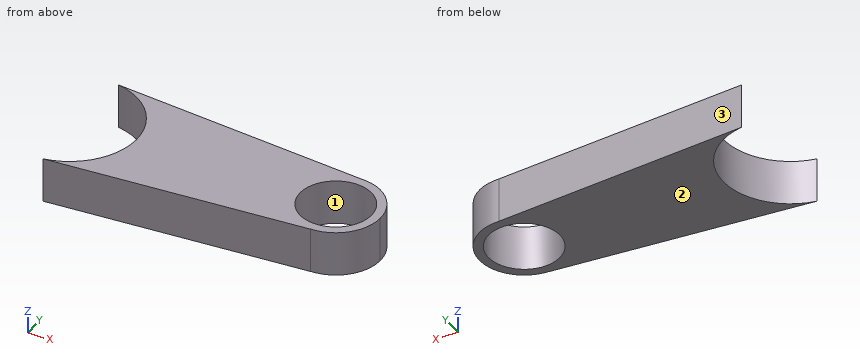
from build123d import *

# Parameters (mm, degrees)
F1_DEPTH = 5
F3_D     = 8


with BuildPart() as f1:
    # F0 (on Top) → F1 (new body)
    with BuildSketch(Plane.XY):
        with BuildLine():
            ThreePointArc((14.5967810947, -5), (18.1323150007, -3.5355339059), (19.5967810947, 0))
            ThreePointArc((19.5967810947, 0), (18.1323150007, 3.5355339059), (14.5967810947, 5))
            Line((14.5967810947, 5), (14.5967810947, 0))
            Line((14.5967810947, 0), (14.5967810947, -5))
        make_face()
        with BuildLine():
            Line((14.5967810947, 0), (14.5967810947, 5))
            ThreePointArc((14.5967810947, 5), (9.5967810947, 0), (14.5967810947, -5))
            Line((14.5967810947, -5), (14.5967810947, 0))
        make_face()
        with BuildLine():
            ThreePointArc((14.5967810947, -5), (9.5967810947, 0), (14.5967810947, 5))
            Line((14.5967810947, 5), (-14.1023044895, 7.3961588722))
            ThreePointArc((-14.1023044895, 7.3961588722), (-9.6198593647, 4.8436616619), (-7.8460222776, 0))
            ThreePointArc((-7.8460222776, 0), (-9.6226170145, -4.8469198667), (-14.110724196, -7.39756978))
            Line((-14.110724196, -7.39756978), (14.5967810947, -5.0171596368))
            Line((14.5967810947, -5.0171596368), (14.5967810947, -5))
        make_face()
    extrude(amount=F1_DEPTH)

    # F3 (through all)
    with Locations(Plane(origin=(0, 0, 0), x_dir=(1, 0, 0), z_dir=(0, 0, -1))):
        with Locations((14.5967810947, 0)):
            Hole(F3_D / 2)


solid = f1.part
Input: part model. Units: mm. Frame: model coordinates. Face numbers are marked on the shaded views. Coordinates: 2 decimals unless noted, no trailing zeros. Loops run counter-clockwise (first coordinate to the right, second up) from the corner with the lowest first, then second, coordinate; pieces in that order, holes last.
Q1. Cut plane D-D (x = 5.5). Output: boundary loops of the cut face in (y, z), then the cut area to 3 significant figures.
Q2. Cut plane A-A (x = -9). Output: boundary loops of the cut face in (y, z).
Q3. Cut plane C-C (y = -3.5). Output: boundary loops of the cut face in (x, z).
Q4. Draft query along X for the marked faces 1, 2 and 3. Return one class per face: +X half, -X half, draft (parallel to the pull), parting line (faces both ways), or undercut.
Q5. Contact query for flat-ended pins moving along their axis: pin 1 (1.5 mm diameter, centred on x = 15.5, z = 2.5, fed in from +Y); pin 2 (1 mm diameter, centred on x = -2.5, z = 3, fed in from -Y); pin 3 (3 mm diameter, centred on x = 4.5, z = 2.5, fed in from -Y). Output: stop coordinate, or through.
Q6. Material intervals for line 1 (X direction, y = -2.5, z = 3.15); line 2 (X direction, y = -1, z = 1.85); line 3 (Y direction, x = -11, z = 1.3), sorted ascending.
Working result:
1. outline: (-5.77, 0) - (5.76, 0) - (5.76, 5) - (-5.77, 5) - close
1. area: 57.7 mm2
2. outline: (-6.97, 0) - (-4, 0) - (-4, 5) - (-6.97, 5) - close; (4, 0) - (6.97, 0) - (6.97, 5) - (4, 5) - close
3. outline: (-8.71, 0) - (12.66, 0) - (12.66, 5) - (-8.71, 5) - close; (16.53, 0) - (18.17, 0) - (18.17, 5) - (16.53, 5) - close
4. face 1: undercut
4. face 2: draft
4. face 3: +X half
5. pin 1: stops at y = 5
5. pin 2: stops at y = -6.48
5. pin 3: stops at y = -5.98
6. line 1: x = -8.27 to 11.47, 17.72 to 18.93
6. line 2: x = -7.91 to 10.72, 18.47 to 19.5
6. line 3: y = -7.14 to -6.11, 6.11 to 7.14
